Verification items for this drawing (mm, ordinates from the low corner). A direction names the side the tool comes from. Round coordinates to 2 decimals unless told otherwise and drop trailing zeros. Order: outer loops, then holes, each group sorted by start corner. A loop starts at its lowest first (then second) coordinate and runs counter-clockwise, first axis right, second up.
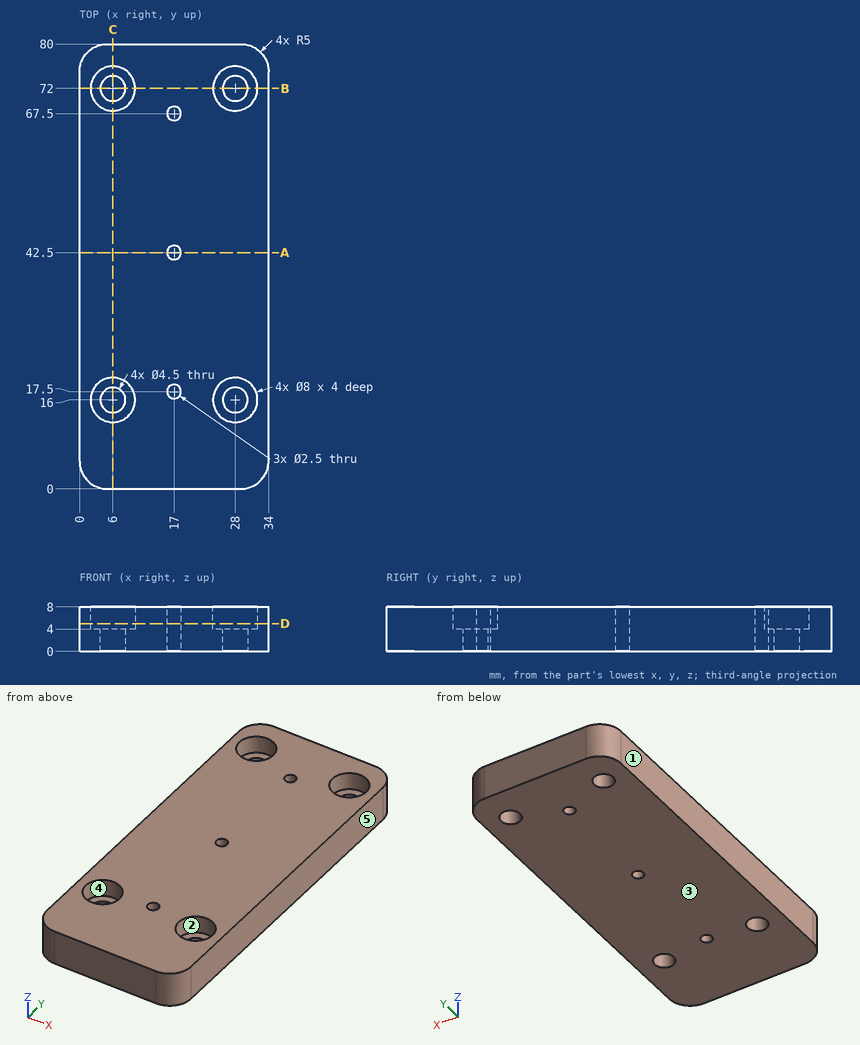
Item 1: Access from +Z, -Z, +X, -X, +Y, -Y to the whole of each face (thin tool, end or side, straight path). Record for the marked faces 1 and 2.
Answer:
face 1: +Z, -Z, -X, +Y, -Y
face 2: +Z
Item 2: Sectioned sample at B-B (y = 72). Record the cut outline in (x, z), and give its area (3 significant figures).
Answer:
outline: (0, 0) - (3.75, 0) - (3.75, 4) - (2, 4) - (2, 8) - (0, 8) - close; (8.25, 0) - (25.75, 0) - (25.75, 4) - (24, 4) - (24, 8) - (10, 8) - (10, 4) - (8.25, 4) - close; (30.25, 0) - (34, 0) - (34, 8) - (32, 8) - (32, 4) - (30.25, 4) - close
area: 172 mm2
Item 3: Sectioned sample at D-D (z = 5). Record the cut outline in (x, y).
Answer:
outline: (0, 5) arc R5 ccw to (5, 0) - (29, 0) arc R5 ccw to (34, 5) - (34, 75) arc R5 ccw to (29, 80) - (5, 80) arc R5 ccw to (0, 75) - close; hole circle Ø8 at (6, 16); hole circle Ø8 at (6, 72); hole circle Ø2.5 at (17, 17.5); hole circle Ø2.5 at (17, 42.5); hole circle Ø2.5 at (17, 67.5); hole circle Ø8 at (28, 16); hole circle Ø8 at (28, 72)
Item 4: Go/stop test with flat-tipped pins: P1, Ø2.5, axis at x = 29, y = 70, coming from the +Z side; P2, Ø4, axis at x = 6, y = 72, coming from the +Z side. Record where each tip stops, or that it passes through.
Answer:
P1: stops at z = 4
P2: passes through
Item 5: Release check for a two-part mould opening along X. For the marked faces 3, 4 and 5 record: released by +X, released by -X, zero draft, split by the parting line, or undercut.
Answer:
face 3: zero draft
face 4: undercut
face 5: released by +X
Item 6: Sectioned sample at A-A (y = 42.5). Record the cut outline in (x, z), and give its area (3 significant figures).
Answer:
outline: (0, 0) - (15.75, 0) - (15.75, 8) - (0, 8) - close; (18.25, 0) - (34, 0) - (34, 8) - (18.25, 8) - close
area: 252 mm2
Item 7: Sectioned sample at C-C (x = 6). Record the cut outline in (y, z).
Answer:
outline: (0, 0) - (13.75, 0) - (13.75, 4) - (12, 4) - (12, 8) - (0, 8) - close; (18.25, 0) - (69.75, 0) - (69.75, 4) - (68, 4) - (68, 8) - (20, 8) - (20, 4) - (18.25, 4) - close; (74.25, 0) - (80, 0) - (80, 8) - (76, 8) - (76, 4) - (74.25, 4) - close
Item 8: Scan lines: line 1 along Y through (x, z) = (28, 6); line 2 along X through (y, z) = (73, 6.25); line 3 along Y through (x, z) = (6, 2.55). Record each from-to range of solid material in increasing order.
Answer:
line 1: y = 0 to 12, 20 to 68, 76 to 80
line 2: x = 0 to 2.13, 9.87 to 24.13, 31.87 to 34
line 3: y = 0 to 13.75, 18.25 to 69.75, 74.25 to 80
